from build123d import *

# Parameters (mm, degrees)
SKETCH_1_R               = 31
EXTRUDE_1_DEPTH          = 6
SKETCH_2_R               = 24
CUT_EXTRUDE_1_DEPTH      = 45.24929378
EXTRUDE_2_DEPTH          = 6
SKETCH_5_R               = 31
SKETCH_5_R_2             = 23
EXTRUDE_3_DEPTH          = 1
HOLE_WIZARD_M3_1_D       = 3.6
PATTERN_CIRCULAR_1_COUNT = 8
HOLE_WIZARD_M3_2_D       = 3.4
PATTERN_CIRCULAR_4_COUNT = 8


with BuildPart() as part:
    # ｽｹｯﾁ1 → ﾎﾞｽ - 押し出し1 (new body)
    with BuildSketch(Plane.XY):
        Circle(SKETCH_1_R)
    extrude(amount=EXTRUDE_1_DEPTH)

    # ｽｹｯﾁ2 → ｶｯﾄ - 押し出し1 (cut, through all)
    with BuildSketch(Plane.XY.offset(6)):
        Circle(SKETCH_2_R)
    extrude(amount=-CUT_EXTRUDE_1_DEPTH, mode=Mode.SUBTRACT)

    # ｽｹｯﾁ3 → ﾎﾞｽ - 押し出し2 (add, through all)
    with BuildSketch(Plane.XY.offset(6)):
        with BuildLine():
            ThreePointArc((-11.41577611, 21.111135825), (-16.970562748, 16.970562748), (-21.111135825, 11.41577611))
            Line((-21.111135825, 11.41577611), (-11.41577611, 21.111135825))
        make_face()
        with BuildLine():
            Line((-11.41577611, -21.111135825), (-21.111135825, -11.41577611))
            ThreePointArc((-21.111135825, -11.41577611), (-16.970562748, -16.970562748), (-11.41577611, -21.111135825))
        make_face()
        with BuildLine():
            ThreePointArc((21.111135825, 11.41577611), (16.970562748, 16.970562748), (11.41577611, 21.111135825))
            Line((11.41577611, 21.111135825), (21.111135825, 11.41577611))
        make_face()
        with BuildLine():
            Line((21.111135825, -11.41577611), (11.41577611, -21.111135825))
            ThreePointArc((11.41577611, -21.111135825), (16.970562748, -16.970562748), (21.111135825, -11.41577611))
        make_face()
    extrude(amount=-EXTRUDE_2_DEPTH)

    # ｽｹｯﾁ5 → ﾎﾞｽ - 押し出し3 (add)
    with BuildSketch(Plane.XY.offset(6)):
        Circle(SKETCH_5_R)
        with Locations(Location((0, 0, 0), (0, 0, 225))):
            Circle(SKETCH_5_R_2, mode=Mode.SUBTRACT)
    extrude(amount=EXTRUDE_3_DEPTH)

    # M3 すきま穴1 (through all)
    with Locations(Plane.XY.offset(7)):
        with Locations((0, 27.5)):
            hole_wizard_m3_1 = Hole(HOLE_WIZARD_M3_1_D / 2)

    # 円形ﾊﾟﾀｰﾝ1: M3 すきま穴1 ×8 about axis
    pattern_circular_1_axis = Axis((0, 0, 0), (0, 0, 1))
    for i in range(1, PATTERN_CIRCULAR_1_COUNT):
        add(hole_wizard_m3_1.rotate(pattern_circular_1_axis, i * 360 / PATTERN_CIRCULAR_1_COUNT), mode=Mode.SUBTRACT)

    # M3 すきま穴2 (through all)
    with Locations(Plane.XY.offset(7)):
        with Locations((10.52379439, 25.406687144)):
            hole_wizard_m3_2 = Hole(HOLE_WIZARD_M3_2_D / 2)

    # 円形ﾊﾟﾀｰﾝ4: M3 すきま穴2 ×8 about axis
    pattern_circular_4_axis = Axis((0, 0, 0), (0, 0, 1))
    for i in range(1, PATTERN_CIRCULAR_4_COUNT):
        add(hole_wizard_m3_2.rotate(pattern_circular_4_axis, i * 360 / PATTERN_CIRCULAR_4_COUNT), mode=Mode.SUBTRACT)


solid = part.part
CAD build for the part. Positions are in the model's coordinates, mm. A direction names the side the tool comes from. Coordinates: 2 decimals unless noted, no trailing zeros. Loops run counter-clockwise (first coordinate to the right, second up) from the corner with the lowest first, then second, coordinate; pieces in that order, holes last. Notation, with made-up numbers: (69.25, 31) - (83.25, 31) arc R8 ccw to (83.25, 37) - close; hole circle Ø3 at (0, 41.5). An arc over 180 degrees is marked (long way). Use one line per item in the form item = value. Start each with the question number.
1) Band-saw the part on D-D (z = 0.75). State how many separate pieces and enclosed holes the cut face has, and give its area (3 significant figures).
2) Two-plate mould, pull along Y, no slides. Class faces 1 (the face through (-23.1, -2.2, 7)), 2 (the face through (-19.368, 21.244, 3.451)): +Y half, -Y half, draft (parallel to the pull), parting line (faces both ways), or undercut.
3) Band-saw the part on A-A (x = 0). Give the cut face in (y, z).
4) Flat gauge pins, fed straight in: pin 1 (3 mm diameter, centred on y = 11, z = 4.5, fed in from +X); pin 2 (1 mm diameter, centred on y = 11.5, z = 5, fed in from +X); pin 3 (8.5 mm diameter, centred on x = 18.5, y = 3.5, fed in from -Z). Where does each tip first touch, or does it go through?
5) Band-saw the part on C-C (x = 6.5). Give the cut face in (y, z), and give its area (3 significant figures).
6) Band-saw the part on B-B (y = 19.5). Give the cut face in (x, z).
7) Drill centre lines: L1, parallel to X at y = -10, z = 4.75; L2, parallel to Y at x = -26.5, z = 2.5; L3, parallel to Y at x = 20, z = 3.5. Where is each one in solid material? Low to high. Write a range as from..to.
8) Tool access for faces 3 (the face through (16.196, 16.331, 3.042)), 4 (the face through (-29.285, 0.234, 3.451)): list every direction of +Z, -Z, +X, -X, +Y, -Y with a clear straight run to the whole face (end or side of a thin tool).
Check values:
q1.separate_pieces = 1
q1.enclosed_holes = 17
q1.area = 1,090 mm2
q2.face_1 = draft
q2.face_2 = undercut
q3.outline = (-31, 0) - (-29.3, 0) - (-29.3, 7) - (-31, 7) - close; (-25.7, 0) - (-24, 0) - (-24, 6) - (-23, 6) - (-23, 7) - (-25.7, 7) - close; (23, 6) - (24, 6) - (24, 0) - (25.7, 0) - (25.7, 7) - (23, 7) - close; (29.3, 0) - (31, 0) - (31, 7) - (29.3, 7) - close
q4.pin_1 = 29.51
q4.pin_2 = 28.98
q4.pin_3 = 6
q5.outline = (-30.31, 0) - (-23.1, 0) - (-23.1, 6) - (-22.06, 6) - (-22.06, 7) - (-30.31, 7) - close; (22.06, 6) - (23.1, 6) - (23.1, 0) - (30.31, 0) - (30.31, 7) - (22.06, 7) - close
q5.area = 103 mm2
q6.outline = (-24.1, 0) - (-21.24, 0) - (-21.24, 7) - (-24.1, 7) - close; (-17.65, 0) - (-13.03, 0) - (-13.03, 6) - (-12.2, 6) - (-12.2, 7) - (-17.65, 7) - close; (12.2, 6) - (13.03, 6) - (13.03, 0) - (17.65, 0) - (17.65, 7) - (12.2, 7) - close; (21.24, 0) - (24.1, 0) - (24.1, 7) - (21.24, 7) - close
q7.L1 = -29.34..-27.02, -23.79..-21.82, 21.82..23.79, 27.02..29.34
q7.L2 = -16.09..-11.83, -9.22..-1.5, 1.5..9.22, 11.83..16.09
q7.L3 = -23.69..-21.16, -17.73..-12.53, 12.53..17.73, 21.16..23.69
q8.face_3 = -Z
q8.face_4 = +Z, -Z
